```python
from build123d import *

# Parameters (mm, degrees)
BOSS_EXTRUDE1_DEPTH = 40
CUT_EXTRUDE1_DEPTH  = 35
BOSS_EXTRUDE2_DEPTH = 5
SKETCH6_R           = 2
CUT_EXTRUDE2_DEPTH  = 70.936511941
SKETCH7_R           = 3.1
SKETCH7_R_2         = 2.1
SKETCH7_R_3         = 2
CUT_EXTRUDE4_DEPTH  = 71.710678119
SKETCH8_R           = 5.05
CUT_EXTRUDE5_DEPTH  = 73.972597597
SKETCH10_W          = 8
SKETCH10_H          = 40
CUT_EXTRUDE8_DEPTH  = 70.936511941


with BuildPart() as part:
    # Sketch1 → Boss-Extrude1 (new body)
    with BuildSketch(Plane(origin=(0, 0, 0), x_dir=(1, 0, 0), z_dir=(0, 1, 0))):
        Polygon((0, 0), (50, 0), (50, 5), (18.181818182, 5), (4.545454545, 18.636363636), (4.545454545, 35), (0, 35), align=None)
    extrude(amount=BOSS_EXTRUDE1_DEPTH)

    # Sketch3 → Cut-Extrude1 (cut)
    with BuildSketch(Plane.XZ):
        Polygon((4.545454545, -18.636363636), (4.545454545, -5), (18.181818182, -5), align=None)
    extrude(amount=-CUT_EXTRUDE1_DEPTH, mode=Mode.SUBTRACT)

    # Sketch5 → Boss-Extrude2 (add)
    with BuildSketch(Plane.XZ):
        Polygon((4.545454545, -20), (4.545454545, -5), (20, -5), align=None)
    extrude(amount=-BOSS_EXTRUDE2_DEPTH)

    # Sketch6 → Cut-Extrude2 (cut, through all)
    with BuildSketch(Plane(origin=(4.545454545, 0, 0), x_dir=(0, 0, -1), z_dir=(1, 0, 0))):
        with Locations((13, 30)):
            Circle(SKETCH6_R)
        with Locations((13, 10)):
            Circle(SKETCH6_R)
        with Locations((21, 20)):
            Circle(SKETCH6_R)
    extrude(amount=-CUT_EXTRUDE2_DEPTH, mode=Mode.SUBTRACT)

    # Sketch7 → Cut-Extrude4 (cut, through all)
    with BuildSketch(Plane(origin=(0, 0, -5), x_dir=(-1, 0, 0), z_dir=(0, 0, -1))):
        with Locations((-35, 12)):
            Circle(SKETCH7_R)
        with Locations((-35, 23)):
            Circle(SKETCH7_R_2)
        with Locations((-25.8, 32)):
            Circle(SKETCH7_R_3)
        with Locations((-44.2, 32)):
            Circle(SKETCH7_R_3)
    extrude(amount=-CUT_EXTRUDE4_DEPTH, mode=Mode.SUBTRACT)

    # Sketch8 → Cut-Extrude5 (cut, through all)
    with BuildSketch(Plane.XY):
        with Locations((35, 12)):
            Circle(SKETCH8_R)
    extrude(amount=-CUT_EXTRUDE5_DEPTH, mode=Mode.SUBTRACT)

    # Sketch10 → Cut-Extrude8 (cut, through all)
    with BuildSketch(Plane(origin=(4.545454545, 0, 0), x_dir=(0, 0, -1), z_dir=(1, 0, 0))):
        with Locations((31, 20)):
            Rectangle(SKETCH10_W, SKETCH10_H)
    extrude(amount=-CUT_EXTRUDE8_DEPTH, mode=Mode.SUBTRACT)


solid = part.part
```
Geometry check sheet. Reference: the model listing, model coordinates, mm. A direction names the side the tool comes from. Give positions to 0.01 mm unless a question says otherwise; leave off trailing zeros. Loops run counter-clockwise (first coordinate to the right, second up) from the corner with the lowest first, then second, coordinate; pieces in that order, holes last. Notation, with made-up numbers: M 18.5,-8 L 29.5,-8 A15 ccw 29.5,-1 Z; hole C -10,35.25 d9. An arc over 180 degrees is marked long. Write item = value, one per line.
(1) Release check for a two-part mould opening along X. For faces 1 (the face through (24.877, 30.226, -2.535)), 2 (the face through (43.277, 30.226, -2.535)), 3 (the face through (0, 20, -14)), 4 (the face through (9, 5, -9)) record: released by +X, released by -X, zero draft, split by the parting line, or undercut.
Answer below:
face_1 = undercut
face_2 = undercut
face_3 = released by -X
face_4 = zero draft
(2) Sectioned sample at B-B, the plane y = 23. Record the cut outline in (x, z).
Answer below:
outline = M 0,-27 L 4.55,-27 L 4.55,-5 L 32.9,-5 L 32.9,0 L 0,0 Z; M 37.1,-5 L 50,-5 L 50,0 L 37.1,0 Z
(3) Sectioned sample at A-A, the plane x = 25.8. Record the cut outline in (y, z), plus the area to 3 significant figures.
Answer below:
outline = M 0,-5 L 30,-5 L 30,0 L 0,0 Z; M 34,-5 L 40,-5 L 40,0 L 34,0 Z
area = 180 mm2
(4) Gauge pin test, flat ends, axial feed: pin 1 Ø3 at (y, z) = (30.5, -9) entering from +X; pin 2 Ø9 at (x, y) = (35, 12) entering from -Z; pin 3 Ø12 at (x, y) = (22, 5) entering from -Z; pin 4 Ø10 at (y, z) = (30, -17) entering from -X. Record the tip position at first contact, or that the pin passes through.
Answer below:
pin_1 = 4.55
pin_2 = through
pin_3 = -8.88
pin_4 = 0
(5) Material ranges on line 1 (Y direction, x = 35, z = -3.05); line 2 (Y direction, x = 25.8, z = -2.7); line 3 (Y direction, x = 3.35, z = -21), recorded low to high. Write a range as [from, to].
Answer below:
line_1 = [0, 6.95], [17.05, 20.9], [25.1, 40]
line_2 = [0, 30], [34, 40]
line_3 = [0, 18], [22, 40]
(6) Sectioned sample at C-C, the plane z = -21. Record the cut outline in (x, y), plus the area to 3 significant figures.
Answer below:
outline = M 0,0 L 4.55,0 L 4.55,18 L 0,18 Z; M 0,22 L 4.55,22 L 4.55,40 L 0,40 Z
area = 164 mm2
(7) Tool access check on faces 5 (the face through (11.46, 37.47, -11.72)), 6 (the face through (28, 20, -5)), 7 (the face through (2, 20, -27)). Record the directions out of +Z, -Z, +X, -X, +Y, -Y that give a thin tool (end or side, any length) a straight path to the whole face; none if there is none.
Answer below:
face_5 = -Z, +X, +Y
face_6 = -Z, +X
face_7 = -Z, +X, -X, +Y, -Y
(8) Sectioned sample at D-D, the plane y = 9. Record the cut outline in (x, z), plus the area to 3 significant figures.
Answer below:
outline = M 0,-27 L 4.55,-27 L 4.55,-14.73 L 0,-14.73 Z; M 0,-11.27 L 4.55,-11.27 L 4.55,-5 L 30.94,-5 L 30.94,0 L 0,0 Z; M 39.06,-5 L 50,-5 L 50,0 L 39.06,0 Z
area = 294 mm2
